Model file for the job. Use its own axes, mm. Face numbers are marked on the shaded views. A direction names the side the tool comes from. Coordinates: 2 decimals unless noted, no trailing zeros. Order: outer loops, then holes, each group sorted by start corner. A loop starts at its lowest first (then second) coordinate and runs counter-clockwise, first axis right, second up.
from build123d import *

# Parameters (mm, degrees)
SKETCH2_W                   = 75
SKETCH2_H                   = 75
BOSS_EXTRUDE1_DEPTH         = 5
SKETCH2_2_W                 = 75
SKETCH2_2_H                 = 75
BOSS_EXTRUDE2_DEPTH         = 5
SKETCH4_W                   = 68
SKETCH4_H                   = 66
CUT_EXTRUDE1_DEPTH          = 5
SKETCH5_W                   = 64
SKETCH5_H                   = 62
CUT_EXTRUDE2_DEPTH          = 5
SKETCH14_W                  = 35.4
SKETCH14_H                  = 35.4
BOSS_EXTRUDE9_DEPTH         = 17.7
SKETCH15_W                  = 25.4
SKETCH15_H                  = 25.4
CUT_EXTRUDE3_DEPTH          = 12.7
SKETCH32_R                  = 3
CUT_EXTRUDE6_DEPTH          = 5
SKETCH16_W                  = 32
SKETCH16_H                  = 44
BOSS_EXTRUDE10_DEPTH        = 5
BOSS_EXTRUDE13_DEPTH        = 2.5
BOSS_EXTRUDE14_DEPTH        = 2.5
SKETCH27_W                  = 5
SKETCH27_H                  = 5
SKETCH27_W_2                = 5.344431893
EYEBOLT_BOLT_SUPPORTS_DEPTH = 2.5
BOSS_EXTRUDE15_DEPTH        = 2.5
BOSS_EXTRUDE16_DEPTH        = 2.5
BOSS_EXTRUDE17_DEPTH        = 2.5
BOSS_EXTRUDE18_DEPTH        = 2.5
SKETCH33_W                  = 6.3
SKETCH33_H                  = 5
SKETCH33_W_2                = 5
SKETCH33_H_2                = 6.3
EYEBOLT_MINI_SUPPORTS_DEPTH = 5
SKETCH34_W                  = 2
SKETCH34_H                  = 62
SKETCH34_H_2                = 61.182345807
CUT_EXTRUDE7_DEPTH          = 5


with BuildPart() as part:
    # Sketch2 → Boss-Extrude1 (new body)
    with BuildSketch(Plane(origin=(0, 0, 0), x_dir=(1, 0, 0), z_dir=(0, 1, 0))):
        Rectangle(SKETCH2_W, SKETCH2_H)
    extrude(amount=BOSS_EXTRUDE1_DEPTH)

    # Sketch2<2> → Boss-Extrude2 (add)
    with BuildSketch(Plane(origin=(0, 0, 0), x_dir=(1, 0, 0), z_dir=(0, 1, 0))):
        Rectangle(SKETCH2_2_W, SKETCH2_2_H)
    extrude(amount=-BOSS_EXTRUDE2_DEPTH)

    # Sketch4 → Cut-Extrude1 (cut)
    with BuildSketch(Plane(origin=(0, 5, 0), x_dir=(1, 0, 0), z_dir=(0, 1, 0))):
        Rectangle(SKETCH4_W, SKETCH4_H)
    extrude(amount=-CUT_EXTRUDE1_DEPTH, mode=Mode.SUBTRACT)

    # Sketch5 → Cut-Extrude2 (cut)
    with BuildSketch(Plane(origin=(0, 0, 0), x_dir=(1, 0, 0), z_dir=(0, 1, 0))):
        Rectangle(SKETCH5_W, SKETCH5_H)
    extrude(amount=-CUT_EXTRUDE2_DEPTH, mode=Mode.SUBTRACT)



with BuildPart() as body_2:
    # Sketch14 → Boss-Extrude9 (new body)
    with BuildSketch(Plane(origin=(0, -50, 0), x_dir=(1, 0, 0), z_dir=(0, 1, 0))):
        Rectangle(SKETCH14_W, SKETCH14_H)
    extrude(amount=BOSS_EXTRUDE9_DEPTH)

    # Sketch15 → Cut-Extrude3 (cut)
    with BuildSketch(Plane.XZ.offset(50)):
        Rectangle(SKETCH15_W, SKETCH15_H)
    extrude(amount=-CUT_EXTRUDE3_DEPTH, mode=Mode.SUBTRACT)

    # Sketch32 → Cut-Extrude6 (cut)
    with BuildSketch(Plane(origin=(0, -32.3, 0), x_dir=(1, 0, 0), z_dir=(0, 1, 0))):
        Circle(SKETCH32_R)
    extrude(amount=-CUT_EXTRUDE6_DEPTH, mode=Mode.SUBTRACT)

    # Sketch27 → Eyebolt Bolt Supports (add)
    with BuildSketch(Plane(origin=(0, -50, 0), x_dir=(-1, 0, 0), z_dir=(0, -1, 0))):
        with Locations((-20.2, 0)):
            Rectangle(SKETCH27_W, SKETCH27_H)
        with Locations((20.2, 0)):
            Rectangle(SKETCH27_W, SKETCH27_H)
        with Locations((-0.172215947, -20.2)):
            Rectangle(SKETCH27_W_2, SKETCH27_H)
        with Locations((0, 20.2)):
            Rectangle(SKETCH27_W, SKETCH27_H)
    extrude(amount=-EYEBOLT_BOLT_SUPPORTS_DEPTH)


with BuildPart() as body_3:
    # Sketch16 → Boss-Extrude10 (new body)
    with BuildSketch(Plane(origin=(0, 45, 0), x_dir=(1, 0, 0), z_dir=(0, 1, 0))):
        Rectangle(SKETCH16_W, SKETCH16_H)
    extrude(amount=-BOSS_EXTRUDE10_DEPTH)


with BuildPart() as part_1:
    add(part.part)

    add(body_3.part)  # Boss-Extrude13 merges body 3
    # Sketch21 → Boss-Extrude13 (add)
    with BuildSketch(Plane.XY):
        Polygon((-34, 5), (-37.5, 5), (-37.5, 21.612086276), (-16, 40), (-10.615074094, 40), (-34, 20), align=None)
        Polygon((37.5, 5), (34, 5), (34, 20), (10.615074094, 40), (16, 40), (37.5, 21.612086276), align=None)
    extrude(amount=BOSS_EXTRUDE13_DEPTH)

    # Sketch21<2> → Boss-Extrude14 (add)
    with BuildSketch(Plane.XY):
        Polygon((-34, 20), (-10.615074094, 40), (-16, 40), (-37.5, 21.612086276), (-37.5, 5), (-34, 5), align=None)
        Polygon((34, 5), (37.5, 5), (37.5, 21.612086276), (16, 40), (10.615074094, 40), (34, 20), align=None)
    extrude(amount=-BOSS_EXTRUDE14_DEPTH)


    add(body_2.part)  # Boss-Extrude15 merges body 2
    # Sketch28 → Boss-Extrude15 (add)
    with BuildSketch(Plane.XY):
        Polygon((22.7, -47.5), (37.5, -5), (32.5, -5), (17.7, -47.5), align=None)
        Polygon((-22.7, -47.5), (-37.5, -5), (-32.5, -5), (-17.7, -47.5), align=None)
    extrude(amount=BOSS_EXTRUDE15_DEPTH)

    # Sketch28<2> → Boss-Extrude16 (add)
    with BuildSketch(Plane.XY):
        Polygon((22.7, -47.5), (37.5, -5), (32.5, -5), (17.7, -47.5), align=None)
        Polygon((-22.7, -47.5), (-37.5, -5), (-32.5, -5), (-17.7, -47.5), align=None)
    extrude(amount=-BOSS_EXTRUDE16_DEPTH)

    # Sketch30 → Boss-Extrude17 (add)
    with BuildSketch(Plane(origin=(0, 0, 0), x_dir=(0, 0, -1), z_dir=(1, 0, 0))):
        Polygon((22.7, -47.5), (37.5, -5), (32.5, -5), (17.7, -47.5), align=None)
        Polygon((-37.5, -5), (-22.7, -47.5), (-17.7, -47.5), (-32.5, -5), align=None)
    extrude(amount=BOSS_EXTRUDE17_DEPTH)

    # Sketch30<2> → Boss-Extrude18 (add)
    with BuildSketch(Plane(origin=(0, 0, 0), x_dir=(0, 0, -1), z_dir=(1, 0, 0))):
        Polygon((22.7, -47.5), (37.5, -5), (32.5, -5), (17.7, -47.5), align=None)
        Polygon((-37.5, -5), (-22.7, -47.5), (-17.7, -47.5), (-32.5, -5), align=None)
    extrude(amount=-BOSS_EXTRUDE18_DEPTH)

    # Sketch33 → Eyebolt Mini Supports (add)
    with BuildSketch(Plane(origin=(0, -32.3, 0), x_dir=(1, 0, 0), z_dir=(0, 1, 0))):
        with Locations((20.85, 0)):
            Rectangle(SKETCH33_W, SKETCH33_H)
        with Locations((0, 20.85)):
            Rectangle(SKETCH33_W_2, SKETCH33_H_2)
        with Locations((-20.85, 0)):
            Rectangle(SKETCH33_W, SKETCH33_H)
        with Locations((0, -20.85)):
            Rectangle(SKETCH33_W_2, SKETCH33_H_2)
    extrude(amount=-EYEBOLT_MINI_SUPPORTS_DEPTH)

    # Sketch34 → Cut-Extrude7 (cut)
    with BuildSketch(Plane(origin=(0, 0, 0), x_dir=(1, 0, 0), z_dir=(0, 1, 0))):
        with Locations((-33, 0)):
            Rectangle(SKETCH34_W, SKETCH34_H)
        with Locations((33, 0.408827097)):
            Rectangle(SKETCH34_W, SKETCH34_H_2)
    extrude(amount=-CUT_EXTRUDE7_DEPTH, mode=Mode.SUBTRACT)


solid = part_1.part
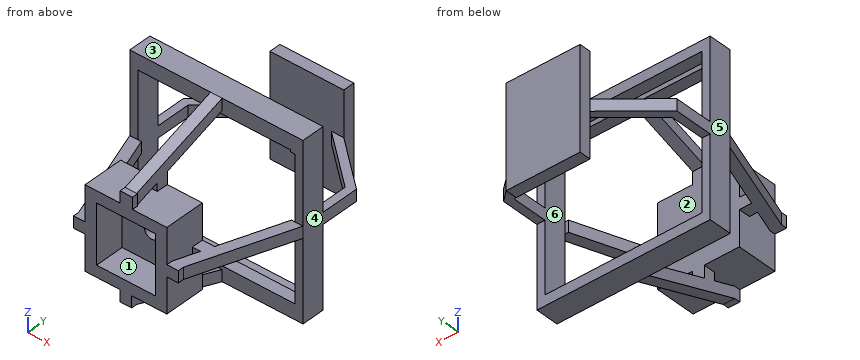
Q1. Mould opens along X. For the marked faces 4, 5 and 6 say: pulls with the +X half, pulls with the -X half, needs draft (parallel to the pull), parting line crosses it, or undercut.
Established:
face 4: pulls with the +X half
face 5: pulls with the -X half
face 6: undercut
Q2. Probe line 1 (X direction, y = 1, z = 23); line 2 (Y direction, x = 8.5, z = -13.5); line 3 (Y direction, x = -7, z = 5). List the from-to ranges inside material, lowest first.
Established:
line 1: x = -37.5 to -34, 34 to 37.5
line 2: y = -50 to -32.3, 40 to 45
line 3: y = -37.3 to -32.3, 40 to 45
Q3. Cut at D-D, the plane y = -26.5. List the corners of the cut face in (x, z).
Established:
outline: (-30.01, -2.5) - (-25.01, -2.5) - (-25.01, 2.5) - (-30.01, 2.5) - close; (-2.5, -30.01) - (2.5, -30.01) - (2.5, -25.01) - (-2.5, -25.01) - close; (-2.5, 25.01) - (2.5, 25.01) - (2.5, 30.01) - (-2.5, 30.01) - close; (25.01, -2.5) - (30.01, -2.5) - (30.01, 2.5) - (25.01, 2.5) - close
Q4. Cut at C-C, the plane x = 0. Count the separate pieces of the cut face and the enclosed holes in it, plus the area to 3 significant figures.
Established:
separate pieces: 3
enclosed holes: 2
area: 1,100 mm2
Q5. Cut at B-B, the plane y = 10.5. List the corners of the cut face in (x, z), plus the area to 3 significant figures.
Established:
outline: (-37.5, -2.5) - (-34, -2.5) - (-34, 2.5) - (-37.5, 2.5) - close; (34, -2.5) - (37.5, -2.5) - (37.5, 2.5) - (34, 2.5) - close
area: 35.0 mm2
Q6. Cut at A-A, the plane y = -42. List the corners of the cut face in (x, z), plus the area to 3 significant figures.
Established:
outline: (-24.62, -2.5) - (-19.62, -2.5) - (-19.62, 2.5) - (-24.62, 2.5) - close; (-17.7, -17.7) - (17.7, -17.7) - (17.7, 17.7) - (-17.7, 17.7) - close; (-2.5, -24.62) - (2.5, -24.62) - (2.5, -19.62) - (-2.5, -19.62) - close; (-2.5, 19.62) - (2.5, 19.62) - (2.5, 24.62) - (-2.5, 24.62) - close; (19.62, -2.5) - (24.62, -2.5) - (24.62, 2.5) - (19.62, 2.5) - close; hole (-12.7, -12.7) - (12.7, -12.7) - (12.7, 12.7) - (-12.7, 12.7) - close
area: 708 mm2
Q7. Which spindle directions (+Z, -Z, +X, -X, +Y, -Y) get a long thin tool onto all of the face, cutting with end or side? Do the marked faces 1, 2 and 3. Say none if no direction does.
Established:
face 1: -Y
face 2: none
face 3: +Z, +X, -X, +Y, -Y
Q8. Drop flat-ended pins along their axis: P1, Ø12, axis at x = 14, y = -27, coming from the +Z side; P2, Ø2.5, axis at x = -7, y = 42.5, coming from the -Z side; P3, Ø16, axis at x = 26.5, y = -21, coming from the +Z side. Give the stop position or say it passes through.
Established:
P1: stops at z = 17.7
P2: stops at z = -22
P3: stops at z = 2.5
